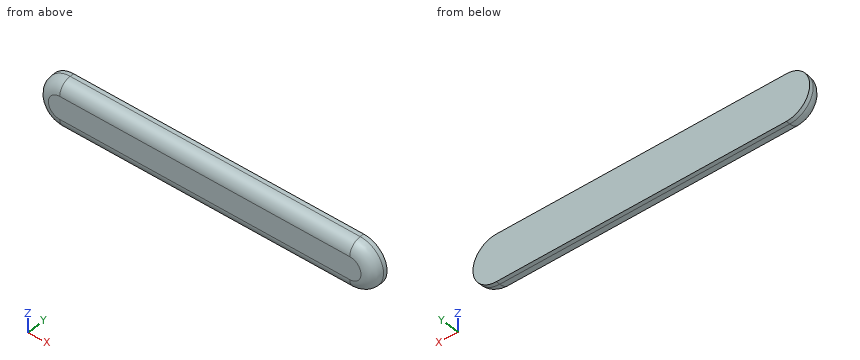
Autodesk Fusion 360 part; units mm, degrees
sketch "SKUF" plane through (0, 0, 0) normal (0, 1, 0) x (1, 0, 0)
  line L0 (-18, 2.9) -> (18, 2.9)
  line L1 (18, 2.9) -> (18, -2.9) construction
  line L2 (18, -2.9) -> (-18, -2.9)
  line L3 (-18, -2.9) -> (-18, 2.9) construction
  arc A0 (-18, 2.9) -> (-18, -2.9) centre (-18, 0) ccw
  arc A1 (18, -2.9) -> (18, 2.9) centre (18, 0) ccw
  line L4 (0, 2.9) -> (0, -2.9) construction
  line L5 (-20.9, 0) -> (20.9, 0) construction
  dimension "d1" = 5.8
  dimension "d2" = 36
  dimension "d10" = 41.6
extrude "Basic shape extrusion" add sketch "SKUF" against normal blind 2
fillet "Bottom fillet" radius 1.5 4 edges at (0, -2, -2.9) (20.9, -2, 0) (0, -2, 2.9) (-20.9, -2, 0)
equation "d1 = SKUF_Z"
equation "d2 = SKUF_X"
equation "d5 = SKUF_STICK_OUT"
equation "SKUF_X = 36 mm"
equation "SKUF_Y = 2.00 mm"
equation "SKUF_Z = 5.80 mm"
equation "SKUF_SLOT_Y = 0.50 mm"
equation "SKUF_STICK_OUT = SKUF_Y - SKUF_SLOT_Y"
properties part number "RW_PARAMETRIC_BUMPON"
For this review, take the finished solid that the model builds, in its own axes (mm). Round coordinates to 2 decimals unless told otherwise and drop trailing zeros. Loops run counter-clockwise (first coordinate to the right, second up) from the corner with the lowest first, then second, coordinate; pieces in that order, holes last.
(1) We need section A-A (x = 15.5). Give the boundary of the cut face in (y, z).
Returned:
outline: (-2, -1.4) arc R1.5 ccw to (-0.5, -2.9) - (0, -2.9) - (0, 2.9) - (-0.5, 2.9) arc R1.5 ccw to (-2, 1.4) - close
(2) Clearance check with a flat-ended pin moving along its axis: P1, Ø1, axis at y = -0.5, z = -1, coming from the +X side. State where the tip first meets the part, or that it passes through.
Returned:
P1: stops at x = 20.86
(3) Wall thickness on line 1 along Y through (x, z) = (6, 2.6); line 2 along Y through (x, z) = (0.5, 1.5); line 3 along Z through (x, y) = (1.5, -1.7): over which ranges is each line inside the solid? List them lowest first.
Returned:
line 1: y = -1.4 to 0
line 2: y = -2 to 0
line 3: z = -2.3 to 2.3
